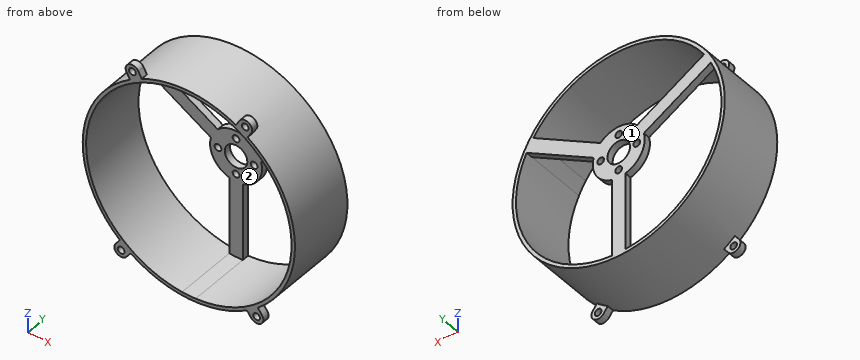
```python
from build123d import *
from build123d.topology import SkipClean

# Parameters (mm, degrees)
SKETCH_1_R          = 47
SKETCH_1_R_2        = 45
EXTRUDE_1_DEPTH     = 30
SKETCH_2_R          = 1.5
EXTRUDE_5_DEPTH     = 3
EXTRUDE_START       = -3
SKETCH_3_R          = 5
SKETCH_3_R_2        = 1.5
EXTRUDE_6_DEPTH     = 3
CUT_EXTRUDE_1_DEPTH = 30
CUT_EXTRUDE_START   = 44
SKETCH_5_R          = 45.5
CUT_EXTRUDE_2_DEPTH = 44


with BuildPart() as part:
    # 草图1 → 凸台-拉伸1 (new body)
    with BuildSketch(Plane(origin=(0, 0, 0), x_dir=(1, 0, 0), z_dir=(0, 1, 0))):
        with Locations(Location((0, 0, 0), (0, 0, 270))):
            Circle(SKETCH_1_R)
        with Locations(Location((0, 0, 0), (0, 0, 270))):
            Circle(SKETCH_1_R_2, mode=Mode.SUBTRACT)
    extrude(amount=EXTRUDE_1_DEPTH)

    # 草图2 → 凸台-拉伸5 (add)
    # profile 1 of 4: a face of its own
    with SkipClean():  # the faces are left unmerged after this step: merging them gives an invalid solid
        with BuildSketch(Plane(origin=(0, 0, 0), x_dir=(-1, 0, 0), z_dir=(0, -1, 0))):
            with BuildLine():
                Line((22.401923789, -44.801270189), (19.851868109, -40.38444419))
                ThreePointArc((19.851868109, -40.38444419), (22.5, -38.97114317), (25.048020532, -37.38444419))
                Line((25.048020532, -37.38444419), (27.598076211, -41.801270189))
                ThreePointArc((27.598076211, -41.801270189), (26.5, -45.899346401), (22.401923789, -44.801270189))
            make_face()
            with Locations(Location((25, -43.301270189, 0), (0, 0, 90))):
                Circle(SKETCH_2_R, mode=Mode.SUBTRACT)
        # profile 2 of 4: a face of its own
        with BuildSketch(Plane(origin=(0, 0, 0), x_dir=(-1, 0, 0), z_dir=(0, -1, 0))):
            with BuildLine():
                Line((-27.598076211, -41.801270189), (-25.048020532, -37.38444419))
                ThreePointArc((-25.048020532, -37.38444419), (-22.5, -38.97114317), (-19.851868109, -40.38444419))
                Line((-19.851868109, -40.38444419), (-22.401923789, -44.801270189))
                ThreePointArc((-22.401923789, -44.801270189), (-26.5, -45.899346401), (-27.598076211, -41.801270189))
            make_face()
            with Locations(Location((-25, -43.301270189, 0), (0, 0, 270))):
                Circle(SKETCH_2_R, mode=Mode.SUBTRACT)
        # profile 3 of 4: a face of its own
        with BuildSketch(Plane(origin=(0, 0, 0), x_dir=(-1, 0, 0), z_dir=(0, -1, 0))):
            with BuildLine():
                Line((32.4, 38.2), (29.339933185, 34.119910913))
                ThreePointArc((29.339933185, 34.119910913), (27, 36), (24.539933185, 37.719910913))
                Line((24.539933185, 37.719910913), (27.6, 41.8))
                ThreePointArc((27.6, 41.8), (31.8, 42.4), (32.4, 38.2))
            make_face()
            with Locations(Location((30, 40, 0), (0, 0, 90))):
                Circle(SKETCH_2_R, mode=Mode.SUBTRACT)
        # profile 4 of 4: a face of its own
        with BuildSketch(Plane(origin=(0, 0, 0), x_dir=(-1, 0, 0), z_dir=(0, -1, 0))):
            with BuildLine():
                Line((-27.6, 41.8), (-24.539933185, 37.719910913))
                ThreePointArc((-24.539933185, 37.719910913), (-27, 36), (-29.339933185, 34.119910913))
                Line((-29.339933185, 34.119910913), (-32.4, 38.2))
                ThreePointArc((-32.4, 38.2), (-31.8, 42.4), (-27.6, 41.8))
            make_face()
            with Locations(Location((-30, 40, 0), (0, 0, 270))):
                Circle(SKETCH_2_R, mode=Mode.SUBTRACT)
        extrude(amount=-EXTRUDE_5_DEPTH)

    # 草图3 → 凸台-拉伸6 (add)
    with SkipClean():  # the faces are left unmerged after this step: merging them gives an invalid solid
        with BuildSketch(Plane(origin=(0, 30, 0), x_dir=(1, 0, 0), z_dir=(0, 1, 0)).offset(EXTRUDE_START)):
            with BuildLine():
                Line((-3, 44.899888641), (-3, 11.101801656))
                ThreePointArc((-3, 11.101801656), (-9.959292144, 5.75), (-11.114442262, -2.952824616))
                Line((-11.114442262, -2.952824616), (-40.38444419, -19.851868109))
                ThreePointArc((-40.38444419, -19.851868109), (-38.97114317, -22.5), (-37.38444419, -25.048020532))
                Line((-37.38444419, -25.048020532), (-8.114442262, -8.148977039))
                ThreePointArc((-8.114442262, -8.148977039), (0, -11.5), (8.114442262, -8.148977039))
                Line((8.114442262, -8.148977039), (37.38444419, -25.048020532))
                ThreePointArc((37.38444419, -25.048020532), (38.97114317, -22.5), (40.38444419, -19.851868109))
                Line((40.38444419, -19.851868109), (11.114442262, -2.952824616))
                ThreePointArc((11.114442262, -2.952824616), (9.959292144, 5.75), (3, 11.101801656))
                Line((3, 11.101801656), (3, 44.899888641))
                ThreePointArc((3, 44.899888641), (0, 45), (-3, 44.899888641))
            make_face()
            with Locations(Location((0, 0, 0), (0, 0, 270))):
                Circle(SKETCH_3_R, mode=Mode.SUBTRACT)
            with Locations(Location((8, 0, 0), (0, 0, 270))):
                Circle(SKETCH_3_R_2, mode=Mode.SUBTRACT)
            with Locations(Location((0, -8, 0), (0, 0, 270))):
                Circle(SKETCH_3_R_2, mode=Mode.SUBTRACT)
            with Locations(Location((-8, 0, 0), (0, 0, 270))):
                Circle(SKETCH_3_R_2, mode=Mode.SUBTRACT)
            with Locations(Location((0, 8, 0), (0, 0, 270))):
                Circle(SKETCH_3_R_2, mode=Mode.SUBTRACT)
        extrude(amount=EXTRUDE_6_DEPTH)

    # 草图4 → 切除-拉伸1 (cut)
    with BuildSketch(Plane.XZ):
        with BuildLine():
            Line((-37.38444419, 25.048020532), (-37.818411718, 25.298571801))
            ThreePointArc((-37.818411718, 25.298571801), (0, 45.5), (37.818411718, 25.298571801))
            Line((37.818411718, 25.298571801), (37.38444419, 25.048020532))
            ThreePointArc((37.38444419, 25.048020532), (0, 45), (-37.38444419, 25.048020532))
        make_face()
        with BuildLine():
            Line((-40.38444419, 19.851868109), (-40.818411718, 20.102419378))
            ThreePointArc((-40.818411718, 20.102419378), (-39.404155872, -22.75), (-3, -45.400991179))
            Line((-3, -45.400991179), (-3, -44.899888641))
            ThreePointArc((-3, -44.899888641), (-38.97114317, -22.5), (-40.38444419, 19.851868109))
        make_face()
        with BuildLine():
            Line((40.38444419, 19.851868109), (40.818411718, 20.102419378))
            ThreePointArc((40.818411718, 20.102419378), (39.404155872, -22.75), (3, -45.400991179))
            Line((3, -45.400991179), (3, -44.899888641))
            ThreePointArc((3, -44.899888641), (38.97114317, -22.5), (40.38444419, 19.851868109))
        make_face()
    extrude(amount=-CUT_EXTRUDE_1_DEPTH, mode=Mode.SUBTRACT)

    # 草图5 → 切除-拉伸2 (cut)
    with SkipClean():  # the faces are left unmerged after this step: merging them gives an invalid solid
        with BuildSketch(Plane(origin=(0, 27, 0), x_dir=(-1, 0, 0), z_dir=(0, -1, 0)).offset(CUT_EXTRUDE_START)):
            with Locations(Location((0, 0, 0), (0, 0, 90))):
                Circle(SKETCH_5_R)
        extrude(amount=-CUT_EXTRUDE_2_DEPTH, mode=Mode.SUBTRACT)


solid = part.part
```
Work out the finished part from the listing and answer in its coordinate system (mm). Face numbers are marked on the shaded views. A direction names the side the tool comes from. Round coordinates to 2 decimals unless told otherwise and drop trailing zeros. Write each loop counter-clockwise with the first axis right and the second up, starting at its lowest first coordinate (ties: lowest second). Pieces come first, ordered by that corner, then holes.
1) A cutting plane is placed at D-D on x = 17. Determine the outline of the cut face in (y, z).
2) Which of the six approach directions +Z, -Z, +X, -X, +Y, -Y give full straight-line access (tool end or side, diameter ignored) to the marked faces 1 and 2?
3) A cutting plane is placed at A-A on z = 0. Determine the outline of the cut face in (x, y), and give its area (3 significant figures).
4) Consider probe 1 along X at (y, z) = (27.85, 0); probe 2 along X at (y, z) = (28, -21); probe 3 along X at (y, z) = (10.25, -0.5). Determine where each line is inside the solid, lowest interval first.
5) A cutting plane is placed at C-C on z = -13.5. Determine the outline of the cut face in (x, y).
6) Flat-ended cylindrical pins translate along their axes: P1, Ø5, axis at x = -25, z = 43.3, coming from the +Y side; P2, Ø3, axis at y = 12, z = 6.5, coming from the +X side; P3, Ø8, axis at x = 37, z = 13, coming from the +Y side; P4, Ø5, axis at x = 8, z = 0, coming from the +Y side. Find the tip coordinate at first contact, or state that the pin passes through.
7) A cutting plane is placed at B-B on y = 13.75. Determine the outline of the cut face in (x, z).
Entries:
1. outline: (0, -43.82) - (30, -43.82) - (30, -42.2) - (0, -42.2) - close; (0, 42.2) - (30, 42.2) - (30, 43.82) - (0, 43.82) - close; (27, 6.35) - (30, 6.35) - (30, 13.28) - (27, 13.28) - close
2. face 1: +Z, -Z, +X, -X, +Y
2. face 2: -Y
3. outline: (-47, 0) - (-45.5, 0) - (-45.5, 30) - (-47, 30) - close; (-11.5, 27) - (-9.5, 27) - (-9.5, 30) - (-11.5, 30) - close; (-6.5, 27) - (-5, 27) - (-5, 30) - (-6.5, 30) - close; (5, 27) - (6.5, 27) - (6.5, 30) - (5, 30) - close; (9.5, 27) - (11.5, 27) - (11.5, 30) - (9.5, 30) - close; (45.5, 0) - (47, 0) - (47, 30) - (45.5, 30) - close
3. area: 111 mm2
4. probe 1: x = -47 to -45.5, -11.5 to -9.5, -6.5 to -5, 5 to 6.5, 9.5 to 11.5, 45.5 to 47
4. probe 2: x = -42.05 to -40.36, -3 to 3, 40.36 to 42.05
4. probe 3: x = -47 to -45.5, 45.5 to 47
5. outline: (-45.02, 0) - (-43.45, 0) - (-43.45, 30) - (-45.02, 30) - close; (-3, 27) - (3, 27) - (3, 30) - (-3, 30) - close; (43.45, 0) - (45.02, 0) - (45.02, 30) - (43.45, 30) - close
6. P1: stops at y = 3
6. P2: stops at x = 46.73
6. P3: passes through
6. P4: stops at y = 30
7. outline: circle Ø94 at (0, 0); hole circle Ø91 at (0, 0)
